Geometry check sheet. Reference: the model listing, model coordinates, mm. Give positions to 0.01 mm unless a question says otherwise; leave off trailing zeros. Order: outer loops, then holes, each group sorted by start corner. A loop starts at its lowest first (then second) coordinate and runs counter-clockwise, first axis right, second up. Notation, with made-up numbers: (68, 11.25) - (99, 11.25) arc R16 ccw to (99, 16.25) - close; hole circle Ø1 at (30, 1). An arc over 180 degrees is marked (long way). Put each result on its own line as item: value. Start each with the question number.
```python
from build123d import *

# Parameters (mm, degrees)
CYLINDER1921_R               = 1.5
CYLINDER1921_DEPTH           = 20
CYLINDER1921_PLACEMENT_ANGLE = 45
CYLINDER1925_R               = 1.5
CYLINDER1925_DEPTH           = 20
CYLINDER1919_R               = 1.5
CYLINDER1919_DEPTH           = 20
CYLINDER1919_PLACEMENT_ANGLE = 135
CYLINDER1920_R               = 1.5
CYLINDER1920_DEPTH           = 20
CYLINDER1922_R               = 1.5
CYLINDER1922_DEPTH           = 20
CYLINDER1922_PLACEMENT_ANGLE = 225
CYLINDER1924_R               = 1.5
CYLINDER1924_DEPTH           = 20
CYLINDER1923_R               = 1.5
CYLINDER1923_DEPTH           = 20
CYLINDER1923_PLACEMENT_ANGLE = 45
CYLINDER1926_R               = 1.5
CYLINDER1926_DEPTH           = 20
CYLINDER1918_R               = 34
CYLINDER1918_DEPTH           = 2


with BuildPart() as obj1:
    # Cylinder1921 → Cylinder1921 (new body)
    with BuildSketch(Plane.XY):
        Circle(CYLINDER1921_R)
    extrude(amount=CYLINDER1921_DEPTH)


with BuildPart() as obj1_1:
    # Cylinder1921 placement: moved
    add(obj1.part.moved(Location((-18.031223, 18.031223, -4))).rotate(Axis((-18.031223, 18.031223, -4), (0, 0, 1)), CYLINDER1921_PLACEMENT_ANGLE))


with BuildPart() as obj2:
    # Cylinder1925 → Cylinder1925 (new body)
    with BuildSketch(Plane(origin=(-25.5, 0, -4), x_dir=(0, 1, 0), z_dir=(0, 0, 1))):
        Circle(CYLINDER1925_R)
    extrude(amount=CYLINDER1925_DEPTH)


with BuildPart() as obj3:
    # Cylinder1919 → Cylinder1919 (new body)
    with BuildSketch(Plane.XY):
        Circle(CYLINDER1919_R)
    extrude(amount=CYLINDER1919_DEPTH)


with BuildPart() as obj3_1:
    # Cylinder1919 placement: moved
    add(obj3.part.moved(Location((-18.031223, -18.031223, -4))).rotate(Axis((-18.031223, -18.031223, -4), (0, 0, 1)), CYLINDER1919_PLACEMENT_ANGLE))


with BuildPart() as obj4:
    # Cylinder1920 → Cylinder1920 (new body)
    with BuildSketch(Plane(origin=(0, -25.5, -4), x_dir=(-1, 0, 0), z_dir=(0, 0, 1))):
        Circle(CYLINDER1920_R)
    extrude(amount=CYLINDER1920_DEPTH)


with BuildPart() as obj5:
    # Cylinder1922 → Cylinder1922 (new body)
    with BuildSketch(Plane.XY):
        Circle(CYLINDER1922_R)
    extrude(amount=CYLINDER1922_DEPTH)


with BuildPart() as obj5_1:
    # Cylinder1922 placement: moved
    add(obj5.part.moved(Location((18.031223, -18.031223, -4))).rotate(Axis((18.031223, -18.031223, -4), (0, 0, 1)), CYLINDER1922_PLACEMENT_ANGLE))


with BuildPart() as obj6:
    # Cylinder1924 → Cylinder1924 (new body)
    with BuildSketch(Plane(origin=(25.5, 0, -4), x_dir=(0, -1, 0), z_dir=(0, 0, 1))):
        Circle(CYLINDER1924_R)
    extrude(amount=CYLINDER1924_DEPTH)


with BuildPart() as obj7:
    # Cylinder1923 → Cylinder1923 (new body)
    with BuildSketch(Plane.XY):
        Circle(CYLINDER1923_R)
    extrude(amount=CYLINDER1923_DEPTH)


with BuildPart() as obj7_1:
    # Cylinder1923 placement: moved
    add(obj7.part.moved(Location((18.031223, 18.031223, -4))).rotate(Axis((18.031223, 18.031223, -4), (0, 0, -1)), CYLINDER1923_PLACEMENT_ANGLE))


with BuildPart() as compound917:
    # Cylinder1926 → Cylinder1926 (new body)
    with BuildSketch(Plane(origin=(0, 25.5, -4), x_dir=(1, 0, 0), z_dir=(0, 0, 1))):
        Circle(CYLINDER1926_R)
    extrude(amount=CYLINDER1926_DEPTH)

    # Compound917: union obj1, obj2, obj3, obj4, obj5, obj6, obj7
    add(obj1_1.part)
    add(obj2.part)
    add(obj3_1.part)
    add(obj4.part)
    add(obj5_1.part)
    add(obj6.part)
    add(obj7_1.part)


with BuildPart() as compound917_1:
    # Compound917 placement: moved
    add(compound917.part.moved(Location((0, 0, 100))))


with BuildPart() as cut564:
    # Cylinder1918 → Cylinder1918 (new body)
    with BuildSketch(Plane.XY.offset(96)):
        Circle(CYLINDER1918_R)
    extrude(amount=CYLINDER1918_DEPTH)

    # Cut564: cut Compound917
    add(compound917_1.part, mode=Mode.SUBTRACT)


with BuildPart() as cut564_1:
    # Cut564 placement: moved
    add(cut564.part.moved(Location((0, 0, 1))))


solid = cut564_1.part
```
Item 1: Thickness scan on line 1 along Y through (x, z) = (0, 98.5); line 2 along X through (y, z) = (18, 97.7); line 3 along Y through (x, z) = (19, 97.8). Record the ranges inside material, lowest first.
Item 2: Cross-section at C-C (z = 97.9). Count the separate pieces of the cut face and the enclosed holes in it, and give its area (3 significant figures).
Item 3: Cross-section at D-D (x = -25.5). Enter the section's corners in (y, z).
Item 4: Cross-section at B-B (y = 18). Enter the section's corners in (x, z), and give its area (3 significant figures).
Item 5: Release check for a two-part mould opening along X. For faces 1 (the face through (0, 0, 97)), 2 (the face through (18.28, 28.67, 97.99)), 3 (the face through (0, 27, 98)) record: +X half, -X half, draft (parallel to the pull), parting line (faces both ways), or undercut.
Item 6: Cross-section at A-A (x = 0). Enter the section's corners in (y, z).
Recorded:
1. line 1: y = -34 to -27, -24 to 24, 27 to 34
1. line 2: x = -28.84 to -19.53, -16.53 to 16.53, 19.53 to 28.84
1. line 3: y = -28.2 to -19.18, -16.89 to 16.89, 19.18 to 28.2
2. separate pieces: 1
2. enclosed holes: 8
2. area: 3,580 mm^2
3. outline: (-22.49, 97) - (-1.5, 97) - (-1.5, 99) - (-22.49, 99) - close; (1.5, 97) - (22.49, 97) - (22.49, 99) - (1.5, 99) - close
4. outline: (-28.84, 97) - (-19.53, 97) - (-19.53, 99) - (-28.84, 99) - close; (-16.53, 97) - (16.53, 97) - (16.53, 99) - (-16.53, 99) - close; (19.53, 97) - (28.84, 97) - (28.84, 99) - (19.53, 99) - close
4. area: 103 mm^2
5. face 1: draft
5. face 2: parting line
5. face 3: undercut
6. outline: (-34, 97) - (-27, 97) - (-27, 99) - (-34, 99) - close; (-24, 97) - (24, 97) - (24, 99) - (-24, 99) - close; (27, 97) - (34, 97) - (34, 99) - (27, 99) - close
